Here's how the part is built. I have some questions about the finished solid (model axes, mm). Face numbers are marked on the shaded views. Give positions to 0.01 mm unless a question says otherwise; leave off trailing zeros. Order: outer loops, then holes, each group sorted by start corner. A loop starts at its lowest first (then second) coordinate and runs counter-clockwise, first axis right, second up. Notation, with made-up numbers: (-15, 17.5) - (-3, 17.5) arc R15 cw to (-3, 43.5) - close; hole circle Ø10 at (-32.5, -7). An arc over 180 degrees is marked (long way). One line per question, with ' | ' between items.
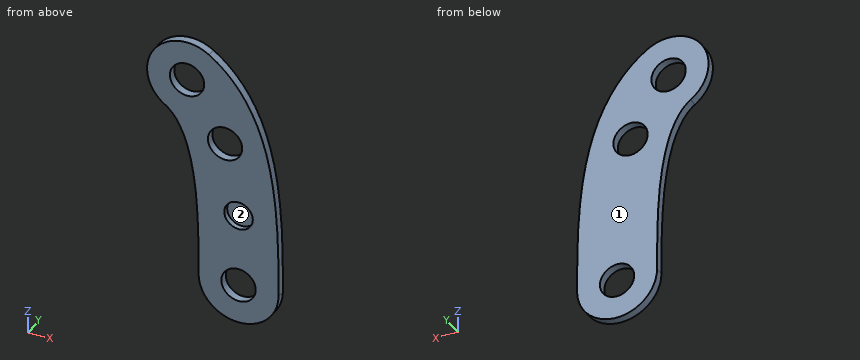
from build123d import *

# Parameters (mm, degrees)
F0_R     = 6
F1_DEPTH = 3
F3_R     = 5.5
F4_DEPTH = 2
F5_R     = 5
F6_DEPTH = 2
F9_ANGLE = 180


# Not quite as in the source:
# - ends of sketch curves that miss each other by under 0.0002 mm in the source are joined
# - the dataset's text gives a spline's control points without its knots; the knots are read off the source's solid


with BuildPart() as f1:
    # F0 (on Front) → F1 (new body)
    with BuildSketch(Plane.XZ):
        with BuildLine():
            add(Edge.make_bspline(
                [(-14, -26), (-14, -22.75), (-14.0004523743, -15.9105291262), (-13.7828666825, -5.0097493319), (-13.1111411806, 6.2097947293), (-11.720563989, 17.4707102353), (-9.6943656003, 26.7000282147), (-7.3231272908, 33.8894297819), (-5.0899646489, 39.15233442), (-2.3107556278, 44.2379137207), (1.1152604329, 49.0651401417), (5.2757801793, 53.5029660938), (8.5623848122, 56.0788774956), (10.3247279458, 57.2378033443)],
                knots=[0, 0, 0, 0, 0.125, 0.25, 0.375, 0.5, 0.625, 0.6875, 0.75, 0.8125, 0.875, 0.9375, 1, 1, 1, 1], degree=3))
            ThreePointArc((-14, -26), (0, -40), (14, -26))
            add(Edge.make_bspline(
                [(14, -26), (14, -22.75), (14.0004523743, -16.1086995406), (14.205139987, -6.0382727532), (14.8002343988, 3.7711749321), (15.9432970346, 12.9047719201), (17.4360428506, 19.5652612944), (18.9356431663, 24.0782015665), (20.186235287, 27.0007682339), (21.5241909854, 29.4228421126), (22.9015337641, 31.3389176928), (24.2833500376, 32.7935083509), (25.2194773121, 33.5209300274), (25.7092571932, 33.8430120472)],
                knots=[0, 0, 0, 0, 0.125, 0.25, 0.375, 0.5, 0.625, 0.6875, 0.75, 0.8125, 0.875, 0.9375, 0.9999998504, 0.9999998504, 0.9999998504, 0.9999998504], degree=3))
            ThreePointArc((25.7092571932, 33.8430120472), (29.7143803557, 53.2326803132), (10.3247279458, 57.2378033443))
        make_face()
        with Locations((0, -26)):
            Circle(F0_R, mode=Mode.SUBTRACT)
        with Locations((4.704827633, 25.5707762288)):
            Circle(F0_R, mode=Mode.SUBTRACT)
        with Locations((18.0169899591, 45.5404115335)):
            Circle(F0_R, mode=Mode.SUBTRACT)
    extrude(amount=F1_DEPTH)


with BuildPart() as f2_1:
    # F2: copy of F1
    add(f1.part.moved(Location((50.8967, 0, 0))))

    # F3 (on face) → F4 (cut)
    with BuildSketch(Plane.XZ.offset(3)):
        with Locations((50.8965918246, 0)):
            Circle(F3_R)
    extrude(amount=-F4_DEPTH, mode=Mode.SUBTRACT)


with BuildPart() as f1_1:
    add(f1.part)

    # F5 (on face) → F6 (cut)
    with BuildSketch(Plane(origin=(0, 0, 0), x_dir=(-1, 0, 0), z_dir=(0, 1, 0))):
        Circle(F5_R)
    extrude(amount=-F6_DEPTH, mode=Mode.SUBTRACT)


with BuildPart() as f1_2:
    # F9: moved
    add(f1_1.part.rotate(Axis((0, 0, 5.4726116359), (0, 0, -1)), F9_ANGLE))


solid = f1_2.part
1) I'm going to push a flat-ended pin straight in: P1, Ø3, axis at x = -1.5, z = -0.5, coming from the -Y side. Where does the tip first touch, or does it pass through?
Model answer:
P1: stops at y = 2
2) I want a section at A-A (z = -28). List the corners of the cut face in (x, y) for me.
Model answer:
outline: (-13.86, 0) - (-5.66, 0) - (-5.66, 3) - (-13.86, 3) - close; (5.66, 0) - (13.86, 0) - (13.86, 3) - (5.66, 3) - close
3) Thinking about a two-plate mould opening in Z: for the marked faces 1 and 2, which applies, +Z half, -Z half, draft (parallel to the pull), parting line (faces both ways), or undercut?
Model answer:
face 1: draft | face 2: undercut
4) I want a section at B-B (x = 0). State how many separate pieces and enclosed holes the cut face has, plus the area to 3 significant figures.
Model answer:
separate pieces: 3 | enclosed holes: 0 | area: 184 mm2
5) Please list where these lines run through material, in increasing order: L1, parallel to X at y = 1.4, z = -25.5; L2, parallel to Z at x = 4, y = 1.35; L3, parallel to Z at x = -4.5, y = 1.3.
Model answer:
L1: x = -14 to -5.98, 5.98 to 14 | L2: z = -39.42 to -30.47, -21.53 to -3, 3 to 41.09 | L3: z = -39.26 to -29.97, -22.03 to -2.18, 2.18 to 19.57, 31.57 to 52.56
